The model under review builds one solid part; all positions refer to its coordinate system, in mm. Round coordinates to 2 decimals unless told otherwise and drop trailing zeros. Write each loop counter-clockwise with the first axis right and the second up, starting at its lowest first coordinate (ties: lowest second). Pieces come first, ordered by that corner, then holes.
Item 1: Clearance check with flat-ended pins moving along their axes: pin 1 Ø16.5 at (x, y) = (-1.5, 7) entering from +Z; pin 2 Ø1.1 at (y, z) = (-11, 0.5) entering from +X; pin 3 Ø1.5 at (y, z) = (11, 1.5) entering from -X; pin 4 Ø2 at (x, y) = (23.055, 0) entering from +Z. State where each tip first meets the part, or that it passes through.
Item 2: Add section C-C (z = 1.75). Give the boundary of the cut face in (x, y) (3 decimals), plus the area to 3 significant figures.
Item 3: To check wall thickness, follow L1, parallel to Y at x = 0, z = 0.45; L2, parallel to Z at x = 6.5, y = 13; L3, parallel to X at y = -1, z = 1.6. State the ranges of each line that lie inside material, in increasing order.
Item 4: Add section B-B (x = -5). Give the boundary of the cut face in (y, z), plus the area to 3 significant figures.
Item 5: Add section A-A (y = 0). Give the boundary of the cut face in (x, z) (3 decimals), plus the area to 3 significant figures.
Item 6: Add section D-D (x = 16.22). Give the boundary of the cut face in (y, z) (3 decimals), plus the area to 3 significant figures.
```python
from build123d import *

# Parameters (mm, degrees)
SKETCH1_R           = 7
BOSS_EXTRUDE1_DEPTH = 1
SKETCH2_R           = 1.485
BOSS_EXTRUDE2_DEPTH = 2
SKETCH2_5_R         = 1.7
CUT_EXTRUDE1_DEPTH  = 32.818104658


with BuildPart() as part:
    # Sketch1 → Boss-Extrude1 (new body)
    with BuildSketch(Plane.XY):
        with BuildLine():
            Line((-9.165, -17.722), (9.165, -17.722))
            Line((9.165, -17.722), (14.25, -13.9625))
            Line((14.25, -13.9625), (14.25, -6.056))
            Line((14.25, -6.056), (24.036185701, -3.112242975))
            ThreePointArc((24.036185701, -3.112242975), (26.349993684, -0.006407429), (24.048450078, 3.108527376))
            Line((24.048450078, 3.108527376), (14.25, 6.098155459))
            ThreePointArc((14.25, 6.098155459), (8.536058528, 12.937762743), (0, 15.5))
            ThreePointArc((0, 15.5), (-8.536058528, 12.937762743), (-14.25, 6.098155459))
            Line((-14.25, 6.098155459), (-24.048450078, 3.108527376))
            ThreePointArc((-24.048450078, 3.108527376), (-26.349993684, -0.006407429), (-24.036185701, -3.112242975))
            Line((-24.036185701, -3.112242975), (-14.25, -6.056))
            Line((-14.25, -6.056), (-14.25, -13.9625))
            Line((-14.25, -13.9625), (-9.165, -17.722))
        make_face()
        Circle(SKETCH1_R, mode=Mode.SUBTRACT)
    extrude(amount=BOSS_EXTRUDE1_DEPTH)

    # Sketch2 → Boss-Extrude2 (add)
    with BuildSketch(Plane.XY.offset(1)):
        with Locations((-16.22, 0)):
            Circle(SKETCH2_R)
        with Locations(Location((16.22, 0, 0), (0, 0, 180))):
            Circle(SKETCH2_R)
    extrude(amount=BOSS_EXTRUDE2_DEPTH)

    # Sketch2_5 → Cut-Extrude1 (cut, through all)
    with BuildSketch(Plane.XY.offset(1)):
        with Locations((-23.055, 0)):
            Circle(SKETCH2_5_R)
        with Locations((23.055, 0)):
            Circle(SKETCH2_5_R)
    extrude(amount=-CUT_EXTRUDE1_DEPTH, mode=Mode.SUBTRACT)


solid = part.part
```
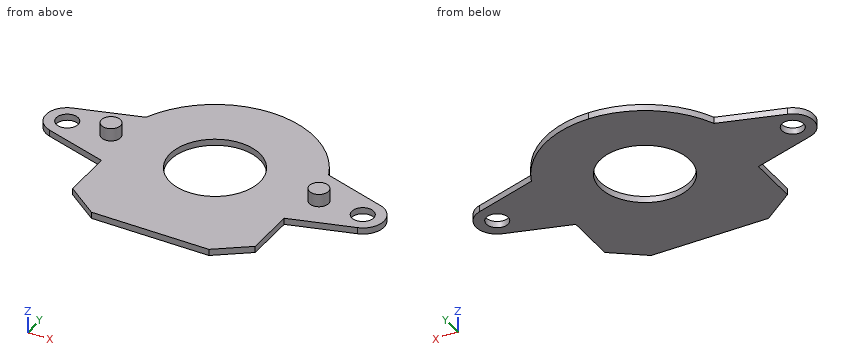
Numbers:
1. pin 1: stops at z = 1
1. pin 2: stops at x = 14.25
1. pin 3: stops at x = -11.46
1. pin 4: passes through
2. outline: circle Ø2.97 at (-16.22, 0); circle Ø2.97 at (16.22, 0)
2. area: 13.9 mm2
3. L1: y = -17.72 to -7, 7 to 15.5
3. L2: z = 0 to 1
3. L3: x = -17.32 to -15.12, 15.12 to 17.32
4. outline: (-17.72, 0) - (-4.9, 0) - (-4.9, 1) - (-17.72, 1) - close; (4.9, 0) - (14.67, 0) - (14.67, 1) - (4.9, 1) - close
4. area: 22.6 mm2
5. outline: (-26.35, 0) - (-24.755, 0) - (-24.755, 1) - (-26.35, 1) - close; (-21.355, 0) - (-7, 0) - (-7, 1) - (-14.735, 1) - (-14.735, 3) - (-17.705, 3) - (-17.705, 1) - (-21.355, 1) - close; (7, 0) - (21.355, 0) - (21.355, 1) - (17.705, 1) - (17.705, 3) - (14.735, 3) - (14.735, 1) - (7, 1) - close; (24.755, 0) - (26.35, 0) - (26.35, 1) - (24.755, 1) - close
5. area: 43.8 mm2
6. outline: (-5.463, 0) - (5.497, 0) - (5.497, 1) - (1.485, 1) - (1.485, 3) - (-1.485, 3) - (-1.485, 1) - (-5.463, 1) - close
6. area: 16.9 mm2
